Design review of the part shown in the three views and the two pictorial views. Dimensions are in mm from the part's minimum x, y and z. A direction names the side the tool comes from. Round coordinates to 2 decimals unless told otherwise and drop trailing zeros. Loops run counter-clockwise (first coordinate to the right, second up) from the corner with the lowest first, then second, coordinate; pieces in that order, holes last. Notation, with made-up numbers: (-13.5, 7) -> (22.5, 7) arc R17 cw to (22.5, 25) -> close; hole circle Ø4 at (81, 42). An arc over 180 degrees is marked (long way). Use a Markdown table: item, result. Add a question column.
1) Insertion check: pin 1 (2 mm diameter, centred on y = 46, z = 14, fed in from -X); pin 2 (4 mm diameter, centred on y = 25, z = 20.5, fed in from -X) (1 decimal); pin 3 (1.5 mm diameter, centred on x = 54.5, z = 8.5, fed in from +Y). Each pin has a flat end and moves straight along its axis. Give the tip position at first contact, or say it passes through.
2) Consider section B-B on y = 29. Give the boundary of the cut face in (x, z) (1 decimal).
3) Consider section A-A on x = 36. Give the boundary of the cut face in (y, z).
4) Consider section D-D on z = 19.5. Give the boundary of the cut face in (x, y) (1 decimal).
5) Wall thickness on probe 1 along X at (y, z) = (52.5, 2.75) (1 decimal); probe 2 along Z at (x, y) = (10.5, 24); probe 3 along Y at (x, z) = (51, 17): over which ranges is each line inside the solid? List them lowest first.
6) For the marked faces 1 and 2, list the 3-axis set-ups (+Z, -Z, +X, -X, +Y, -Y) from which the entire face can be reached by the end or side of a thin tool; tool diameter is ignored.
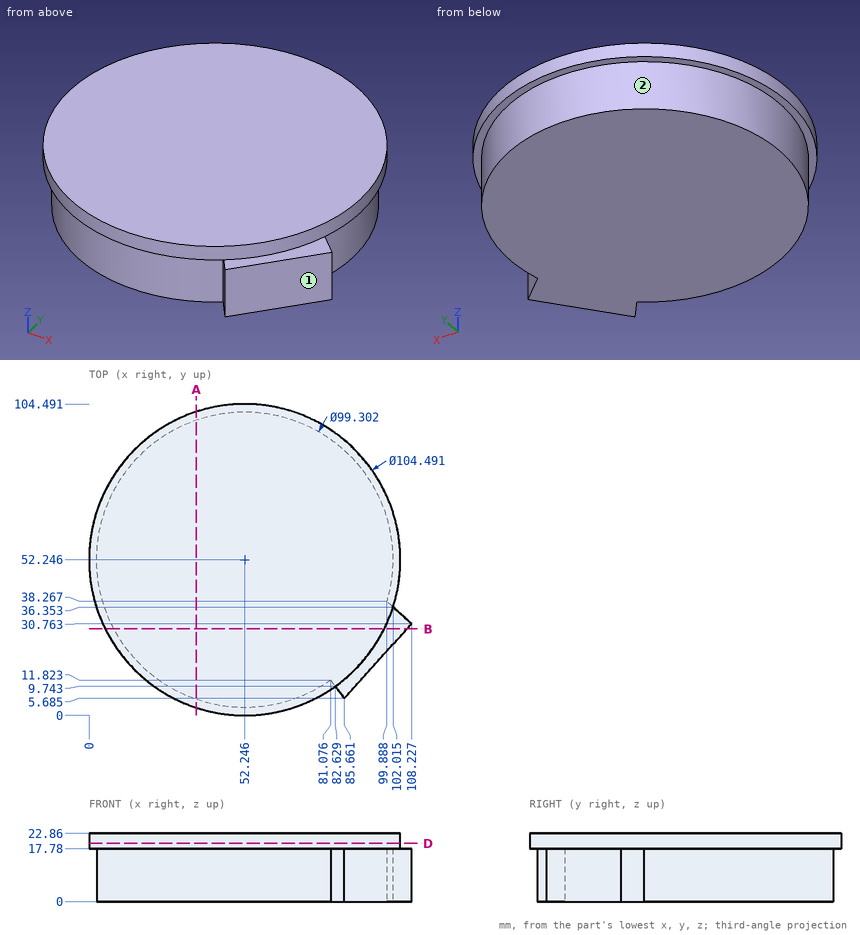
Result set:
| question | item | result |
|---|---|---|
| 1 | pin 1 | x = 2.87 |
| 1 | pin 2 | x = 6.5 |
| 1 | pin 3 | y = 101.87 |
| 2 | outline | (5.5, 17.8) -> (8.4, 17.8) -> (8.4, 0) -> (106.6, 0) -> (106.6, 17.8) -> (99, 17.8) -> (99, 22.9) -> (5.5, 22.9) -> close |
| 3 | outline | (2.59, 17.78) -> (5.33, 17.78) -> (5.33, 0) -> (99.16, 0) -> (99.16, 17.78) -> (101.9, 17.78) -> (101.9, 22.86) -> (2.59, 22.86) -> close |
| 4 | outline | circle Ø104.5 at (52.2, 52.2) |
| 5 | probe 1 | 2.6 to 101.9 |
| 5 | probe 2 | 17.78 to 22.86 |
| 5 | probe 3 | 2.61 to 101.88 |
| 6 | face 1 | +Z, -Z, +X, -Y |
| 6 | face 2 | -Z |
